The model under review builds one solid part; all positions refer to its coordinate system, in mm. Face numbers are marked on the shaded views. A direction names the side the tool comes from. Give positions to 0.01 mm unless a question says otherwise; leave off trailing zeros. Loops run counter-clockwise (first coordinate to the right, second up) from the corner with the lowest first, then second, coordinate; pieces in that order, holes last. Notation, with made-up numbers: (53.25, 16.25) - (107.25, 16.25) arc R19 cw to (107.25, 27.25) - close; hole circle Ø4 at (25.5, 86). An arc over 180 degrees is marked (long way). Return JSON: item names as keys, results as strings. Group by question number.
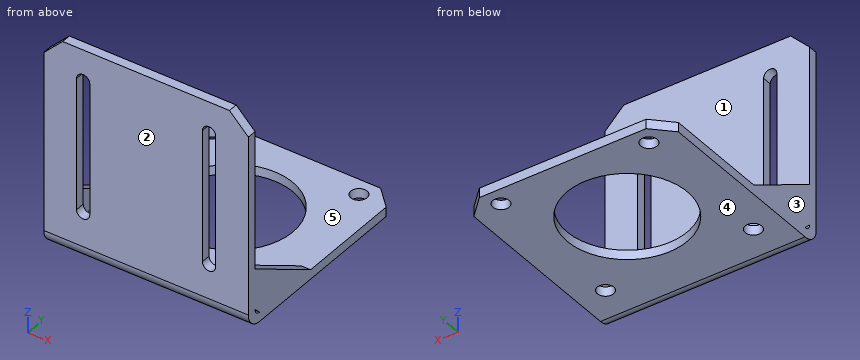
from build123d import *

# Parameters (mm, degrees)
SKETCH1_R           = 19.1
SKETCH1_R_2         = 2.6
BOSS_EXTRUDE1_DEPTH = 3
SKETCH2_W           = 68
SKETCH2_H           = 3
BOSS_EXTRUDE2_DEPTH = 65
BOSS_EXTRUDE3_DEPTH = 3
BOSS_EXTRUDE4_DEPTH = 3
CUT_EXTRUDE1_DEPTH  = 3
CUT_EXTRUDE2_DEPTH  = 65


with BuildPart() as part:
    # Sketch1 → Boss-Extrude1 (new body)
    with BuildSketch(Plane.XY):
        Polygon((-32.5, 59), (-32.5, 0), (32.5, 0), (32.5, 59), (26.5, 65), (-26.5, 65), align=None)
        with Locations((0, 36)):
            Circle(SKETCH1_R, mode=Mode.SUBTRACT)
        with Locations((-23.5, 59.5)):
            Circle(SKETCH1_R_2, mode=Mode.SUBTRACT)
        with Locations((23.5, 59.5)):
            Circle(SKETCH1_R_2, mode=Mode.SUBTRACT)
        with Locations((23.5, 12.5)):
            Circle(SKETCH1_R_2, mode=Mode.SUBTRACT)
        with Locations((-23.5, 12.5)):
            Circle(SKETCH1_R_2, mode=Mode.SUBTRACT)
    extrude(amount=BOSS_EXTRUDE1_DEPTH)

    # Sketch2 → Boss-Extrude2 (add)
    with BuildSketch(Plane.ZY.offset(32.5)):
        with Locations((34, -1.5)):
            Rectangle(SKETCH2_W, SKETCH2_H)
    extrude(amount=-BOSS_EXTRUDE2_DEPTH)

    # Sketch3 → Boss-Extrude3 (add)
    with BuildSketch(Plane.ZY.offset(32.5)):
        Polygon((3, 25), (18, 0), (3, 0), align=None)
    extrude(amount=-BOSS_EXTRUDE3_DEPTH)

    # Sketch4 → Boss-Extrude4 (add)
    with BuildSketch(Plane(origin=(32.5, 0, 0), x_dir=(0, 0, -1), z_dir=(1, 0, 0))):
        Polygon((-3, 0), (-18, 0), (-3, 25), align=None)
    extrude(amount=-BOSS_EXTRUDE4_DEPTH)

    # Sketch5 → Cut-Extrude1 (cut)
    with BuildSketch(Plane(origin=(0, 0, 0), x_dir=(1, 0, 0), z_dir=(0, 1, 0))):
        Polygon((-32.5, -68), (-32.5, -62), (-26.5, -68), align=None)
        Polygon((32.5, -68), (32.5, -62), (26.5, -68), align=None)
        with BuildLine():
            Line((17.9, -58), (17.9, -16))
            ThreePointArc((17.9, -16), (20, -13.9), (22.1, -16))
            Line((22.1, -16), (22.1, -58))
            ThreePointArc((22.1, -58), (20, -60.1), (17.9, -58))
        make_face()
        with BuildLine():
            Line((-22.1, -58), (-22.1, -16))
            ThreePointArc((-22.1, -16), (-20, -13.9), (-17.9, -16))
            Line((-17.9, -16), (-17.9, -58))
            ThreePointArc((-17.9, -58), (-20, -60.1), (-22.1, -58))
        make_face()
    extrude(amount=-CUT_EXTRUDE1_DEPTH, mode=Mode.SUBTRACT)

    # Sketch6 → Cut-Extrude2 (cut)
    with BuildSketch(Plane.ZY.offset(32.5)):
        with BuildLine():
            Line((0, -3), (5, -3))
            ThreePointArc((5, -3), (1.464466094, -1.535533906), (0, 2))
            Line((0, 2), (0, -3))
        make_face()
        with BuildLine():
            Line((3.002550682, 2), (5.002550682, 0))
            ThreePointArc((5.002550682, 0), (3.58833712, 0.585786438), (3.002550682, 2))
        make_face()
    extrude(amount=-CUT_EXTRUDE2_DEPTH, mode=Mode.SUBTRACT)


solid = part.part
Item 1: Take a section at C-C (z = 44.5). State the section outline as (x, y) points, then the cut area to 3 significant figures.
Item 2: For L1, parallel to X at y = 12, z = 1; L2, parallel to Y at x = -23, z = 1; L3, parallel to Y at x = -23.5, z = 1.75, list the stretches that pass through material, from the lowest coordinate up. Write a range as from..to.
Item 3: Tool access review of the marked faces 1 and 2: name each direction out of +Z, -Z, +X, -X, +Y, -Y from which nothing blocks a thin tool from reaching the whole face with its end or side.
Item 4: Take a section at A-A (x = 0). State the section outline as (y, z) points.
Item 5: Take a section at D-D (y = 13.5). State the section outline as (x, z) points, then the cut area to 3 significant figures.
Item 6: Take a section at B-B (y = 36). State the section outline as (x, z) points, then the cut area to 3 significant figures.
Item 7: For P1, Ø19.5, axis at x = 7.5, y = 25, coming from the +Z side; P2, Ø8, axis at x = 25, z = 38, coming from the +Y side, all flat-tipped, find the tip position at first contact; note any pin that passes through.
Item 8: Mouldability with a two-part tool opening along Z and no side actions: class the marked faces 3, 4 and 5 as +Z half, -Z half, draft (parallel to the pull), parting line (faces both ways), or undercut.
Check sheet entries:
{
 "1": {"outline": "(-32.5, -3) - (-22.1, -3) - (-22.1, 0) - (-32.5, 0) - close; (-17.9, -3) - (17.9, -3) - (17.9, 0) - (-17.9, 0) - close; (22.1, -3) - (32.5, -3) - (32.5, 0) - (22.1, 0) - close", "area": "170 mm^2"},
 "2": {"L1": "x = -32.5..-26.05, -20.95..20.95, 26.05..32.5", "L2": "y = -1..9.95, 15.05..56.95, 62.05..65", "L3": "y = -1.8..9.9, 15.1..56.9, 62.1..65"},
 "3": {"face 1": "+Z, +Y", "face 2": "+Z, -Z, +X, -X, -Y"},
 "4": {"outline": "(-3, 5) arc R5 ccw to (2, 0) - (16.9, 0) - (16.9, 3) - (0, 3) - (0, 68) - (-3, 68) - close; (55.1, 0) - (65, 0) - (65, 3) - (55.1, 3) - close"},
 "5": {"outline": "(-32.5, 0) - (-25.9, 0) - (-25.9, 3) - (-29.5, 3) - (-29.5, 9.9) - (-32.5, 9.9) - close; (-21.1, 0) - (21.1, 0) - (21.1, 3) - (-21.1, 3) - close; (25.9, 0) - (32.5, 0) - (32.5, 9.9) - (29.5, 9.9) - (29.5, 3) - (25.9, 3) - close", "area": "208 mm^2"},
 "6": {"outline": "(-32.5, 0) - (-19.1, 0) - (-19.1, 3) - (-32.5, 3) - close; (19.1, 0) - (32.5, 0) - (32.5, 3) - (19.1, 3) - close", "area": "80.4 mm^2"},
 "7": {"P1": "stops at z = 3", "P2": "stops at y = 0"},
 "8": {"face 3": "draft", "face 4": "-Z half", "face 5": "+Z half"}
}
